```python
from build123d import *

# Parameters (mm, degrees)
IZIM1_W                          = 37
IZIM1_H                          = 1.524
IZIM2_W                          = 3
IZIM2_H                          = 42.6
Y_KSEKLIK_EKSTR_ZYON1_DEPTH      = 16.276
IZIM3_W                          = 3
IZIM3_H                          = 42.6
Y_KSEKLIK_EKSTR_ZYON2_DEPTH      = 16.276
DELIK1_D                         = 2.95656
DELIK1_DEPTH                     = 1.524
F_0_15_0_15_DIAMETER_HOLE1_D     = 15
F_0_15_0_15_DIAMETER_HOLE1_DEPTH = 17.8
IZIM15_W                         = 33
IZIM15_H                         = 48.693516851
KES_EKSTR_ZYON2_DEPTH            = 16.276
IZIM16_W                         = 42.6
IZIM16_H                         = 16.276
Y_KSEKLIK_EKSTR_ZYON3_DEPTH      = 1.5
IZIM17_W                         = 42.6
IZIM17_H                         = 16.276
Y_KSEKLIK_EKSTR_ZYON4_DEPTH      = 1.5
IZIM18_W                         = 42.6
IZIM18_H                         = 1.7
Y_KSEKLIK_EKSTR_ZYON5_DEPTH      = 3
IZIM19_W                         = 42.6
IZIM19_H                         = 1.7
Y_KSEKLIK_EKSTR_ZYON6_DEPTH      = 3
IZIM20_R                         = 13
KES_EKSTR_ZYON3_DEPTH            = 39
IZIM21_R                         = 1.25
KES_EKSTR_ZYON4_DEPTH            = 39


with BuildPart() as part:
    # Çizim1 → Döndür1 (revolve)
    with BuildSketch(Plane(origin=(0, 0, 0), x_dir=(-1, 0, 0), z_dir=(0, 0, -1))):
        with Locations((-18.5, 0.762)):
            Rectangle(IZIM1_W, IZIM1_H)
    revolve(axis=Axis((0, 0, 0), (0, 1, 0)))

    # Çizim2 → Yükseklik-Ekstrüzyon1 (add)
    with BuildSketch(Plane(origin=(0, 1.524, 0), x_dir=(-1, 0, 0), z_dir=(0, 1, 0))):
        with Locations((16.5, -0.7)):
            Rectangle(IZIM2_W, IZIM2_H)
    extrude(amount=Y_KSEKLIK_EKSTR_ZYON1_DEPTH)

    # Çizim3 → Yükseklik-Ekstrüzyon2 (add)
    with BuildSketch(Plane(origin=(0, 1.524, 0), x_dir=(-1, 0, 0), z_dir=(0, 1, 0))):
        with Locations((-16.5, -0.7)):
            Rectangle(IZIM3_W, IZIM3_H)
    extrude(amount=Y_KSEKLIK_EKSTR_ZYON2_DEPTH)

    # Delik1
    with Locations(Plane(origin=(0, 1.524, 0), x_dir=(1, 0, 0), z_dir=(0, 1, 0))):
        with Locations((0, 30.48), (30.016940312, 5.292796455), (26.396454307, -15.24), (10.424773969, -28.641831082), (-10.424773969, -28.641831082), (-26.396454307, -15.24), (-30.016940312, 5.292796455)):
            Hole(DELIK1_D / 2, depth=DELIK1_DEPTH)

    # Ø0.15 (0.15) Diameter Hole1
    with Locations(Plane(origin=(0, 0, 0), x_dir=(-1, 0, 0), z_dir=(0, -1, 0))):
        with Locations((0, 0)):
            Hole(F_0_15_0_15_DIAMETER_HOLE1_D / 2, depth=F_0_15_0_15_DIAMETER_HOLE1_DEPTH)

    # Çizim15 → Kes-Ekstrüzyon2 (cut)
    with BuildSketch(Plane(origin=(0, 17.8, 0), x_dir=(1, 0, 0), z_dir=(0, 1, 0))):
        with Locations((0, 0.128603458)):
            Rectangle(IZIM15_W, IZIM15_H)
    extrude(amount=-KES_EKSTR_ZYON2_DEPTH, mode=Mode.SUBTRACT)

    # Çizim16 → Yükseklik-Ekstrüzyon3 (add)
    with BuildSketch(Plane(origin=(18, 0, 0), x_dir=(0, 0, -1), z_dir=(1, 0, 0))):
        with Locations((0.7, 9.662)):
            Rectangle(IZIM16_W, IZIM16_H)
    extrude(amount=Y_KSEKLIK_EKSTR_ZYON3_DEPTH)

    # Çizim17 → Yükseklik-Ekstrüzyon4 (add)
    with BuildSketch(Plane.ZY.offset(18)):
        with Locations((-0.7, 9.662)):
            Rectangle(IZIM17_W, IZIM17_H)
    extrude(amount=Y_KSEKLIK_EKSTR_ZYON4_DEPTH)

    # Çizim18 → Yükseklik-Ekstrüzyon5 (add)
    with BuildSketch(Plane.ZY.offset(19.5)):
        with Locations((-0.7, 18.65)):
            Rectangle(IZIM18_W, IZIM18_H)
    extrude(amount=-Y_KSEKLIK_EKSTR_ZYON5_DEPTH)

    # Çizim19 → Yükseklik-Ekstrüzyon6 (add)
    with BuildSketch(Plane(origin=(19.5, 0, 0), x_dir=(0, 0, -1), z_dir=(1, 0, 0))):
        with Locations((0.7, 18.65)):
            Rectangle(IZIM19_W, IZIM19_H)
    extrude(amount=-Y_KSEKLIK_EKSTR_ZYON6_DEPTH)

    # Çizim20 → Kes-Ekstrüzyon3 (cut)
    with BuildSketch(Plane.ZY.offset(19.5)):
        with Locations((-13.6, 30.5)):
            Circle(IZIM20_R)
    extrude(amount=-KES_EKSTR_ZYON3_DEPTH, mode=Mode.SUBTRACT)

    # Çizim21 → Kes-Ekstrüzyon4 (cut)
    with BuildSketch(Plane.ZY.offset(19.5)):
        with Locations((17.15, 17)):
            Circle(IZIM21_R)
        with Locations((9.15, 17)):
            Circle(IZIM21_R)
        with Locations((1.15, 17)):
            Circle(IZIM21_R)
        with Locations((-6.85, 17)):
            Circle(IZIM21_R)
    extrude(amount=-KES_EKSTR_ZYON4_DEPTH, mode=Mode.SUBTRACT)


solid = part.part
```
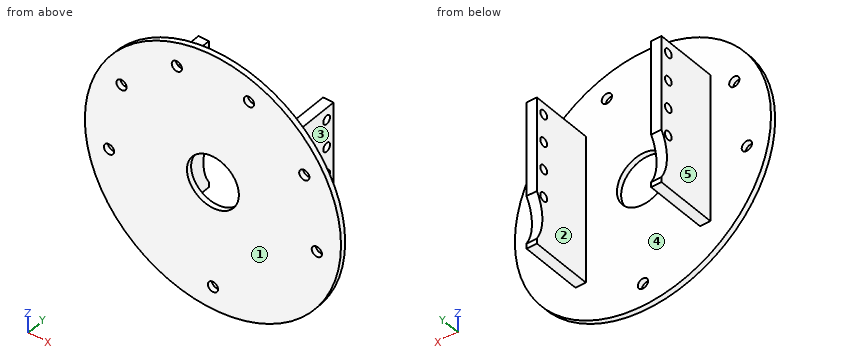
Check sheet for the modelled part. Datum: model origin and axes. Units: mm. Face numbers are marked on the shaded views. A direction names the side the tool comes from. Round coordinates to 2 decimals unless told otherwise and drop trailing zeros. Write each loop counter-clockwise with the first axis right and the second up, starting at its lowest first coordinate (ties: lowest second). Pieces come first, ordered by that corner, then holes. Notation, with made-up numbers: (63.25, -35.5) -> (94.25, -35.5) arc R25 cw to (94.25, -7.5) -> close; hole circle Ø11 at (-28.75, 1). An arc over 180 degrees is marked (long way). Put each result on its own line as item: value.
(1) Go/stop test with flat-tipped pins: pin 1 Ø9 at (y, z) = (13.5, 0) entering from -X; pin 2 Ø9 at (y, z) = (11, -2) entering from +X; pin 3 Ø4 at (x, z) = (11.5, 7) entering from +Y; pin 4 Ø2.5 at (x, z) = (10.42, 28.64) entering from +Y. Record where each tip stops, or that it passes through.
Values found:
pin 1: stops at x = -19.5
pin 2: stops at x = 19.5
pin 3: stops at y = 1.52
pin 4: passes through
(2) Sectioned sample at C-C (z = -30.48). Enter the section's corners in (x, y), plus the area to 3 significant figures.
Values found:
outline: (-20.98, 0) -> (-1.48, 0) -> (-1.48, 1.52) -> (-20.98, 1.52) -> close; (1.48, 0) -> (20.98, 0) -> (20.98, 1.52) -> (1.48, 1.52) -> close
area: 59.4 mm^2
(3) Sectioned sample at A-A (y = 14.5). Enter the section's corners in (x, z), plus the area to 3 significant figures.
Values found:
outline: (-19.5, -22) -> (-16.5, -22) -> (-16.5, 20.6) -> (-19.5, 20.6) -> close; (16.5, -22) -> (19.5, -22) -> (19.5, 20.6) -> (16.5, 20.6) -> close
area: 256 mm^2
(4) Tool access check on the marked faces 1 and 2. Record the directions out of +Z, -Z, +X, -X, +Y, -Y that give a thin tool (end or side, any length) a straight path to the whole face; none if there is none.
Values found:
face 1: +Z, -Z, +X, -X, -Y
face 2: +Z, -Z, +Y
(5) Sectioned sample at B-B (z = 4). Enter the section's corners in (x, y), plus the area to 3 significant figures.
Values found:
outline: (-36.78, 0) -> (-6.34, 0) -> (-6.34, 1.52) -> (-16.5, 1.52) -> (-16.5, 19.5) -> (-19.5, 19.5) -> (-19.5, 1.52) -> (-36.78, 1.52) -> close; (6.34, 0) -> (36.78, 0) -> (36.78, 1.52) -> (19.5, 1.52) -> (19.5, 19.5) -> (16.5, 19.5) -> (16.5, 1.52) -> (6.34, 1.52) -> close
area: 201 mm^2
(6) Material ranges on line 1 (Y direction, x = 18, z = 17); line 2 (X direction, y = 4.5, z = -8); line 3 (Z direction, x = 17, y = 16), recorded low to high.
Values found:
line 1: y = 0 to 15.76, 18.24 to 19.5
line 2: x = -19.5 to -16.5, 16.5 to 19.5
line 3: z = -22 to -7.6, -6.1 to 0.4, 1.9 to 8.4, 9.9 to 16.4, 17.9 to 20.6
(7) Mould release check, pull along X, two halves, no side actions. Record for the marked faces 3, 4 and 5: released by +X, released by -X, zero draft, split by the parting line, or undercut.
Values found:
face 3: released by +X
face 4: undercut
face 5: released by -X
(8) Sectioned sample at D-D (x = -23). Enter the section's corners in (y, z), plus the area to 3 significant figures.
Values found:
outline: (0, -28.98) -> (1.52, -28.98) -> (1.52, 28.98) -> (0, 28.98) -> close
area: 88.3 mm^2
